Can you work these out from the model? Positions are in its coordinate system, mm. A direction names the side the tool comes from. Coordinates: 2 decimals unless noted, no trailing zeros. Order: outer loops, then holes, each group sorted by start corner. A loop starts at its lowest first (then second) coordinate and runs counter-clockwise, first axis right, second up. Notation, with made-up numbers: (-27.5, 44) -> (2.5, 44) arc R25 ccw to (2.5, 74) -> close; hole circle Ø8 at (31, 7.5). An arc over 180 degrees is marked (long way). Return JSON: item names as keys, results as strings. Group by question number.
1) For pin 1 (2 mm diameter, centred on x = 11.5, y = 2, fed in from -Z); pin 2 (12 mm diameter, centred on x = 13, z = 4, fed in from -Y); pin 3 (2 mm diameter, centred on x = 16.5, y = 0.5, fed in from -Z); pin 4 (6 mm diameter, centred on y = -2.5, z = -10.5, fed in from +X), each with a flat end and sliding along its axis, tell me the tip position at first contact or that it passes through.
2) If we section it at B-B, the plane x = 0: Please give me the cut outline in (y, z).
3) If we section it at A-A, the plane z = 0: Please give me the cut outline in (x, y), then the cut area to 4 significant figures.
4) For faces 1 (the cylindrical face through (-0.8, 1.4, -4.5)), 2 (the cylindrical face through (-9.76, -2.46, 2.17)), which set-ups out of +Z, -Z, +X, -X, +Y, -Y let a thin tool reach every point of the face, with its end or its side?
5) If we section it at D-D, the plane z = 12.5: Please give me the cut outline in (x, y).
6) Thinking about a two-plate mould opening in X: for faces 3 (the cylindrical face through (0.9, 1.42, 2.86)), 4 (the flat face through (-5, 5, 10)), 5 (the cylindrical face through (9.76, 6.52, 2.17)), which applies, +X half, -X half, draft (parallel to the pull), parting line (faces both ways), or undercut?
7) If I drill on probe 1 along Y at (x, z) = (16.5, -1.5); probe 2 along X at (y, z) = (7, 1); probe 3 along X at (y, z) = (1.75, 1), over which ranges is the centre line in solid material (lowest first)? Write a range as from..to.
8) If we section it at C-C, the plane x = 14.5: Please give me the cut outline in (y, z), then the cut area to 3 significant figures.
from build123d import *

# Parameters (mm, degrees)
SKETCH_1_R               = 22.5
EXTRUDE_1_DEPTH          = 5
SKETCH_2_R               = 10
EXTRUDE_2_DEPTH          = 5
EXTRUDE_START            = 3
SKETCH_4_R               = 10
EXTRUDE_3_DEPTH          = 3
CUT_EXTRUDE_2_DEPTH      = 35.372954485
CUT_EXTRUDE_2_DEPTH_BACK = 35.372954485
SKETCH_5_R               = 3
HOLE_WIZARD_M4_3_D       = 3.3
SKETCH_10_R              = 2
CUT_EXTRUDE_3_DEPTH      = 35.372954485
CHAMFER_2_SIZE           = 0.5
CHAMFER_4_SIZE           = 0.3


with BuildPart() as part:
    # Sketch 1 → Extrude 1 (new body)
    with BuildSketch(Plane(origin=(0, 0, 0), x_dir=(1, 0, 0), z_dir=(0, 1, 0))):
        with Locations(Location((0, 0, 0), (0, 0, 270))):
            Circle(SKETCH_1_R)
    extrude(amount=EXTRUDE_1_DEPTH)

    # Sketch 2 → Extrude 2 (add)
    with BuildSketch(Plane.XZ):
        with Locations(Location((0, 0, 0), (0, 0, 270))):
            Circle(SKETCH_2_R)
    extrude(amount=EXTRUDE_2_DEPTH)

    # Sketch 4 → Extrude 3 (add)
    with BuildSketch(Plane(origin=(0, 5, 0), x_dir=(1, 0, 0), z_dir=(0, 1, 0)).offset(EXTRUDE_START)):
        with Locations(Location((0, 0, 0), (0, 0, 90))):
            Circle(SKETCH_4_R)
    extrude(amount=-EXTRUDE_3_DEPTH)

    # Sketch 5 → Cut-Extrude 2 (cut, two sides: drawn at the far end of the back side and taken through both)
    with BuildSketch(Plane(origin=(0, 8, 0), x_dir=(1, 0, 0), z_dir=(0, 1, 0)).offset(-CUT_EXTRUDE_2_DEPTH_BACK)):
        with Locations(Location((0, 0, 0), (0, 0, 270))):
            Circle(SKETCH_5_R)
    extrude(amount=CUT_EXTRUDE_2_DEPTH + CUT_EXTRUDE_2_DEPTH_BACK, mode=Mode.SUBTRACT)

    # Hole Wizard M4 _3 (through all)
    with Locations(Plane.XZ):
        with Locations((11.913336036, -13.493421527), (13.493421527, 11.913336036), (-11.913336036, 13.493421527), (-13.493421527, -11.913336036)):
            Hole(HOLE_WIZARD_M4_3_D / 2)

    # Sketch 10 → Cut-Extrude 3 (cut, through all)
    with BuildSketch(Plane(origin=(0, 8, 0), x_dir=(1, 0, 0), z_dir=(0, 1, 0))):
        with Locations(Location((0, 6.332219822, 0), (0, 0, 270))):
            Circle(SKETCH_10_R)
    extrude(amount=-CUT_EXTRUDE_3_DEPTH, mode=Mode.SUBTRACT)

    # Chamfer 2
    chamfer_2_edges = [part.edges().sort_by_distance(p)[0] for p in [
        (0, 8, -3),
        (0, -5, -3),
    ]]
    chamfer(chamfer_2_edges, length=CHAMFER_2_SIZE)

    # Chamfer 4
    chamfer_4_edges = [part.edges().sort_by_distance(p)[0] for p in [
        (0, 8, -8.332219822),
    ]]
    chamfer(chamfer_4_edges, length=CHAMFER_4_SIZE)


solid = part.part
Result sheet:
{
 "1": {"pin 1": "stops at z = -19.9", "pin 2": "stops at y = -5", "pin 3": "stops at z = -16.31", "pin 4": "stops at x = 20.69"},
 "2": {"outline": "(-5, -10) -> (0, -10) -> (0, -22.5) -> (5, -22.5) -> (5, -10) -> (8, -10) -> (8, -8.63) -> (7.7, -8.33) -> (-5, -8.33) -> close; (-5, -4.33) -> (7.7, -4.33) -> (8, -4.03) -> (8, -3.5) -> (7.5, -3) -> (-4.5, -3) -> (-5, -3.5) -> close; (-5, 3.5) -> (-4.5, 3) -> (7.5, 3) -> (8, 3.5) -> (8, 10) -> (5, 10) -> (5, 22.5) -> (0, 22.5) -> (0, 10) -> (-5, 10) -> close"},
 "3": {"outline": "(-22.5, 0) -> (-10, 0) -> (-10, -5) -> (-3.5, -5) -> (-3, -4.5) -> (-3, 7.5) -> (-3.5, 8) -> (-10, 8) -> (-10, 5) -> (-22.5, 5) -> close; (3, -4.5) -> (3.5, -5) -> (10, -5) -> (10, 0) -> (22.5, 0) -> (22.5, 5) -> (10, 5) -> (10, 8) -> (3.5, 8) -> (3, 7.5) -> close", "area": "306.5 mm2"},
 "4": {"face 1": "+Y, -Y", "face 2": "-Y"},
 "5": {"outline": "(-18.71, 0) -> (-13.23, 0) -> (-13.23, 5) -> (-18.71, 5) -> close; (-10.6, 0) -> (11.95, 0) -> (11.95, 5) -> (-10.6, 5) -> close; (15.04, 0) -> (18.71, 0) -> (18.71, 5) -> (15.04, 5) -> close"},
 "6": {"face 3": "undercut", "face 4": "draft", "face 5": "parting line"},
 "7": {"probe 1": "y = 0..5", "probe 2": "x = -9.95..-2.83, 2.83..9.95", "probe 3": "x = -22.48..-2.83, 2.83..22.48"},
 "8": {"outline": "(0, -17.2) -> (5, -17.2) -> (5, 10.61) -> (0, 10.61) -> close; (0, 13.22) -> (5, 13.22) -> (5, 17.2) -> (0, 17.2) -> close", "area": "159 mm2"}
}
